Could you check a few things on this model? Use its own coordinates, in mm. A direction names the side the tool comes from. Round coordinates to 2 decimals unless told otherwise and drop trailing zeros. Order: outer loops, then holes, each group sorted by start corner. A loop starts at its lowest first (then second) coordinate and runs counter-clockwise, first axis right, second up. Notation, with made-up numbers: (24, 41.5) -> (61, 41.5) arc R16 cw to (61, 49.5) -> close; hole circle Ø4 at (77.5, 89.5). An arc over 180 degrees is marked (long way). One line per question, with ' | ' between items.
```python
from build123d import *

# Parameters (mm, degrees)
SKETCH2_W               = 127
SKETCH2_H               = 50.8
BOSS_EXTRUDE1_DEPTH     = 38.1
SKETCH4_W               = 27.94
SKETCH4_H               = 25.4
CUT_EXTRUDE1_DEPTH      = 26.4
CUT_EXTRUDE1_DEPTH_BACK = 26.4
SKETCH5_W               = 30.48
SKETCH5_H               = 12.7
CUT_EXTRUDE2_DEPTH      = 64.5
CUT_EXTRUDE2_DEPTH_BACK = 64.5
BOSS_EXTRUDE2_START     = -50.8
BOSS_EXTRUDE2_DEPTH     = 35.56


with BuildPart() as part:
    # Sketch2 → Boss-Extrude1 (new body)
    with BuildSketch(Plane(origin=(0, 0, 0), x_dir=(1, 0, 0), z_dir=(0, 1, 0))):
        Rectangle(SKETCH2_W, SKETCH2_H)
    extrude(amount=BOSS_EXTRUDE1_DEPTH)

    # Sketch4 → Cut-Extrude1 (cut, two sides)
    with BuildSketch(Plane.XY) as cut_extrude1_sk:
        with Locations((-26.67, 12.7)):
            Rectangle(SKETCH4_W, SKETCH4_H)
        with Locations((26.67, 12.7)):
            Rectangle(SKETCH4_W, SKETCH4_H)
    extrude(amount=CUT_EXTRUDE1_DEPTH, mode=Mode.SUBTRACT)
    extrude(cut_extrude1_sk.sketch, amount=-CUT_EXTRUDE1_DEPTH_BACK, mode=Mode.SUBTRACT)

    # Sketch5 → Cut-Extrude2 (cut, two sides)
    with BuildSketch(Plane(origin=(0, 0, 0), x_dir=(0, 0, -1), z_dir=(1, 0, 0))) as cut_extrude2_sk:
        with Locations((0, 13.97)):
            Rectangle(SKETCH5_W, SKETCH5_H)
    extrude(amount=CUT_EXTRUDE2_DEPTH, mode=Mode.SUBTRACT)
    extrude(cut_extrude2_sk.sketch, amount=-CUT_EXTRUDE2_DEPTH_BACK, mode=Mode.SUBTRACT)

    # Sketch7 → Boss-Extrude2 (add)
    with BuildSketch(Plane(origin=(0, 0, -25.4), x_dir=(-1, 0, 0), z_dir=(0, 0, -1)).offset(BOSS_EXTRUDE2_START)):
        Polygon((48.26, 38.1), (48.26, 63.5), (33.02, 63.5), (33.02, 50.8), (15.24, 50.8), (15.24, 38.1), align=None)
        Polygon((-15.24, 38.1), (-48.26, 38.1), (-48.26, 63.5), (-33.02, 63.5), (-33.02, 50.8), (-15.24, 50.8), align=None)
    extrude(amount=BOSS_EXTRUDE2_DEPTH)


solid = part.part
```
1. I want a section at C-C on x = 46.5. List the corners of the cut face in (y, z) for me.
From the geometry:
outline: (0, -25.4) -> (38.1, -25.4) -> (38.1, -10.16) -> (63.5, -10.16) -> (63.5, 25.4) -> (0, 25.4) -> close; hole (7.62, -15.24) -> (20.32, -15.24) -> (20.32, 15.24) -> (7.62, 15.24) -> close
2. If we mould it in two halves opening along Z, with no side actions, what happens to faces 6 (the face through (0, 14, 15.24)), 7 (the face through (-1, 24, 25.4)), 8 (the face through (-35, 48, -10.16)), 9 (the face through (-52, 0, 0))? For each: pulls with the +Z half, pulls with the -Z half, needs draft (parallel to the pull), parting line crosses it, or undercut.
From the geometry:
face 6: undercut | face 7: pulls with the +Z half | face 8: pulls with the -Z half | face 9: needs draft
3. I want a section at B-B on z = -12. List the corners of the cut face in (x, y) for me.
From the geometry:
outline: (-63.5, 0) -> (-40.64, 0) -> (-40.64, 7.62) -> (-63.5, 7.62) -> close; (-63.5, 20.32) -> (-40.64, 20.32) -> (-40.64, 25.4) -> (-12.7, 25.4) -> (-12.7, 20.32) -> (12.7, 20.32) -> (12.7, 25.4) -> (40.64, 25.4) -> (40.64, 20.32) -> (63.5, 20.32) -> (63.5, 38.1) -> (-63.5, 38.1) -> close; (-12.7, 0) -> (12.7, 0) -> (12.7, 7.62) -> (-12.7, 7.62) -> close; (40.64, 0) -> (63.5, 0) -> (63.5, 7.62) -> (40.64, 7.62) -> close
4. I want a section at A-A on y = 11. List the corners of the cut face in (x, z) for me, and give its area (3 significant figures).
From the geometry:
outline: (-63.5, -25.4) -> (-40.64, -25.4) -> (-40.64, -15.24) -> (-63.5, -15.24) -> close; (-63.5, 15.24) -> (-40.64, 15.24) -> (-40.64, 25.4) -> (-63.5, 25.4) -> close; (-12.7, -25.4) -> (12.7, -25.4) -> (12.7, -15.24) -> (-12.7, -15.24) -> close; (-12.7, 15.24) -> (12.7, 15.24) -> (12.7, 25.4) -> (-12.7, 25.4) -> close; (40.64, -25.4) -> (63.5, -25.4) -> (63.5, -15.24) -> (40.64, -15.24) -> close; (40.64, 15.24) -> (63.5, 15.24) -> (63.5, 25.4) -> (40.64, 25.4) -> close | area: 1,450 mm²
5. I'm going to push flat-ended pins straight in: pin 1 (8 mm diameter, centred on x = 27.5, y = 55, fed in from -Z); pin 2 (6.5 mm diameter, centred on y = 45.5, z = 3.5, fed in from +X); pin 3 (12.5 mm diameter, centred on x = -27.5, y = 49, fed in from -Z); pin 4 (5.5 mm diameter, centred on x = -20, z = 10, fed in from +Y). Where does each tip first touch, or does it pass through?
From the geometry:
pin 1: passes through | pin 2: stops at x = 48.26 | pin 3: stops at z = -10.16 | pin 4: stops at y = 50.8
6. I want a section at D-D on y = 58.5. List the corners of the cut face in (x, z) for me.
From the geometry:
outline: (-48.26, -10.16) -> (-33.02, -10.16) -> (-33.02, 25.4) -> (-48.26, 25.4) -> close; (33.02, -10.16) -> (48.26, -10.16) -> (48.26, 25.4) -> (33.02, 25.4) -> close
7. I need wall thicknesses on probe 1 along X at (y, z) = (4.5, -21); probe 2 along Y at (x, z) = (-58, -6); probe 3 along X at (y, z) = (40, 20). Which ranges of each line are inside material? Lowest first, please.
From the geometry:
probe 1: x = -63.5 to -40.64, -12.7 to 12.7, 40.64 to 63.5 | probe 2: y = 0 to 7.62, 20.32 to 38.1 | probe 3: x = -48.26 to -15.24, 15.24 to 48.26
8. On a 3-axis mill with a long thin cutter (end or side, diameter ignored), from which of +Z, -Z, +X, -X, +Y, -Y can I reach the whole of each face in a straight line? I mean faces 1 (the face through (-27, 25.4, 0)), 2 (the face through (35, 48, -10.16)), 3 (the face through (15.24, 45, 8)), 4 (the face through (52, 20.32, 0)), 5 (the face through (-48.26, 51, 8)). Say none if no direction works.
From the geometry:
face 1: +Z, -Z, -Y | face 2: -Z, +X, -X, +Y | face 3: +Z, -Z, +Y | face 4: +X, -X | face 5: +Z, -Z, -X, +Y
